Part model, mm, in its own coordinate system. Coordinates: 2 decimals unless noted, no trailing zeros. Order: outer loops, then holes, each group sorted by start corner. A loop starts at its lowest first (then second) coordinate and runs counter-clockwise, first axis right, second up. Notation, with made-up numbers: (80.5, 30) - (134.5, 30) arc R26 ccw to (134.5, 57) - close; hole circle Ø3 at (57.25, -17.75). An arc over 180 degrees is marked (long way). Use a Markdown table: item, result. Add a question column.
1) Saw through at B-B on z = -19.5. List the corners of the cut face in (x, y).
2) Saw through at C-C on x = -20. List the corners of the cut face in (y, z), then the cut area to 3 significant figures.
3) Saw through at A-A on y = 4. List the corners of the cut face in (x, z), then the cut area to 3 significant figures.
4) Wall check: L1, parallel to Z at x = 1, y = 24.5; L2, parallel to X at y = 8, z = -25; L3, parallel to X at y = 3.5, z = -30.5. Give the ranges that are in metal, low to high. Write a range as [from, to].
5) Drop flat-ended pins along their axis: P1, Ø10, axis at x = -1.5, y = 8, coming from the -Z side; P2, Ø12, axis at x = -19, y = 24.5, coming from the -Z side; P3, Ø2, axis at y = 12.5, z = -10.5, coming from the +X side; P4, Ø6, axis at x = -22, y = 24, coming from the +Z side. Give the stop position or say it passes through.
```python
from build123d import *

# Parameters (mm, degrees)
SKETCH1_R           = 37
BOSS_EXTRUDE1_DEPTH = 30
CUT_EXTRUDE1_DEPTH  = 30


with BuildPart() as part:
    # Sketch1 → Boss-Extrude1 (new body)
    with BuildSketch(Plane(origin=(0, 0, 0), x_dir=(1, 0, 0), z_dir=(0, 1, 0))):
        Circle(SKETCH1_R)
    extrude(amount=BOSS_EXTRUDE1_DEPTH)

    # Sketch2 → Cut-Extrude1 (cut)
    with BuildSketch(Plane(origin=(0, 30, 0), x_dir=(1, 0, 0), z_dir=(0, 1, 0))):
        with BuildLine():
            Line((6.424982574, 36.437886861), (6.077686218, 34.468271355))
            ThreePointArc((6.077686218, 34.468271355), (24.748737342, 24.748737342), (34.468271355, 6.077686218))
            Line((34.468271355, 6.077686218), (36.437886861, 6.424982574))
            ThreePointArc((36.437886861, 6.424982574), (26.162950904, 26.162950904), (6.424982574, 36.437886861))
        make_face()
        with BuildLine():
            Line((36.437886861, -6.424982574), (34.468271355, -6.077686218))
            ThreePointArc((34.468271355, -6.077686218), (24.748737342, -24.748737342), (6.077686218, -34.468271355))
            Line((6.077686218, -34.468271355), (6.424982574, -36.437886861))
            ThreePointArc((6.424982574, -36.437886861), (26.162950904, -26.162950904), (36.437886861, -6.424982574))
        make_face()
        with BuildLine():
            Line((-6.424982574, -36.437886861), (-6.077686218, -34.468271355))
            ThreePointArc((-6.077686218, -34.468271355), (-24.748737342, -24.748737342), (-34.468271355, -6.077686218))
            Line((-34.468271355, -6.077686218), (-36.437886861, -6.424982574))
            ThreePointArc((-36.437886861, -6.424982574), (-26.162950904, -26.162950904), (-6.424982574, -36.437886861))
        make_face()
        with BuildLine():
            Line((-36.437886861, 6.424982574), (-34.468271355, 6.077686218))
            ThreePointArc((-34.468271355, 6.077686218), (-24.748737342, 24.748737342), (-6.077686218, 34.468271355))
            Line((-6.077686218, 34.468271355), (-6.424982574, 36.437886861))
            ThreePointArc((-6.424982574, 36.437886861), (-26.162950904, 26.162950904), (-36.437886861, 6.424982574))
        make_face()
    extrude(amount=-CUT_EXTRUDE1_DEPTH, mode=Mode.SUBTRACT)


solid = part.part
```
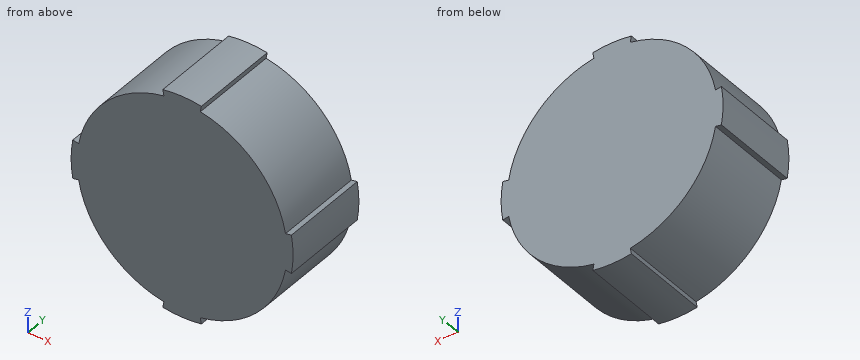
Results are:
| question | item | result |
|---|---|---|
| 1 | outline | (-29.06, 0) - (29.06, 0) - (29.06, 30) - (-29.06, 30) - close |
| 2 | outline | (0, -28.72) - (30, -28.72) - (30, 28.72) - (0, 28.72) - close |
| 2 | area | 1,720 mm2 |
| 3 | outline | (-36.44, -6.42) - (-34.47, -6.08) arc R35 ccw to (-6.08, -34.47) - (-6.42, -36.44) arc R37 ccw to (6.42, -36.44) - (6.08, -34.47) arc R35 ccw to (34.47, -6.08) - (36.44, -6.42) arc R37 ccw to (36.44, 6.42) - (34.47, 6.08) arc R35 ccw to (6.08, 34.47) - (6.42, 36.44) arc R37 ccw to (-6.42, 36.44) - (-6.08, 34.47) arc R35 ccw to (-34.47, 6.08) - (-36.44, 6.42) arc R37 ccw to start |
| 3 | area | 3,950 mm2 |
| 4 | L1 | [-36.99, 36.99] |
| 4 | L2 | [-24.49, 24.49] |
| 4 | L3 | [-17.17, 17.17] |
| 5 | P1 | z = -37 |
| 5 | P2 | z = -32.5 |
| 5 | P3 | x = 33.69 |
| 5 | P4 | z = 29.39 |
